For this review, use the dimensioned drawing (mm, ordinates from the lowest corner) and the shaded views. Coordinates: 2 decimals unless noted, no trailing zeros. Write each loop counter-clockwise with the first axis right and the second up, starting at its lowest first coordinate (ties: lowest second). Pieces come first, ordered by that corner, then holes. Notation, with made-up numbers: (41.25, 74.25) - (81.25, 74.25) arc R29 cw to (81.25, 103.25) - close; hole circle Ø9 at (9, 82). An arc over 180 degrees is marked (long way). One line per item, written item: value.
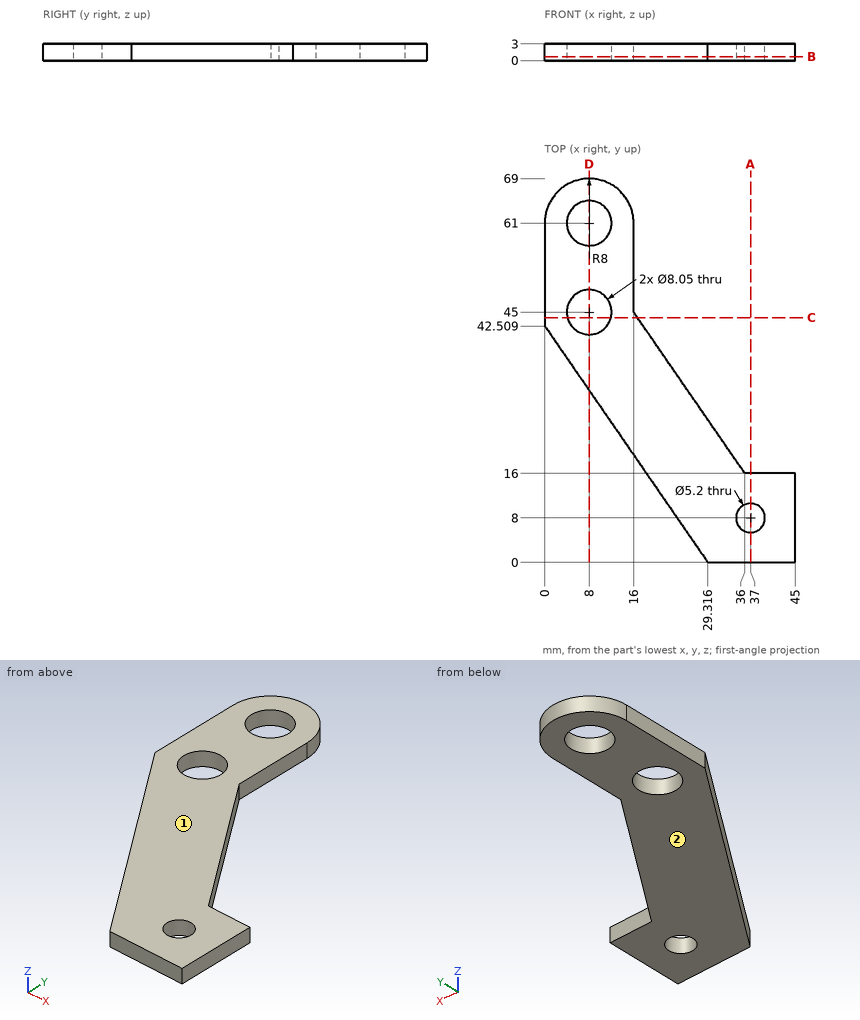
1. Consider section A-A, the plane x = 37. Write out the cut boundary in (y, z), then the cut area to 3 significant figures.
Answer block:
outline: (0, 0) - (5.4, 0) - (5.4, 3) - (0, 3) - close; (10.6, 0) - (16, 0) - (16, 3) - (10.6, 3) - close
area: 32.4 mm^2
2. Consider section D-D, the plane x = 8. Write out the cut boundary in (y, z) (1 decimal).
Answer block:
outline: (30.9, 0) - (41, 0) - (41, 3) - (30.9, 3) - close; (49, 0) - (57, 0) - (57, 3) - (49, 3) - close; (65, 0) - (69, 0) - (69, 3) - (65, 3) - close
3. Insertion check: pin 1 Ø1.5 at (x, z) = (27, 1) entering from +Y; pin 2 Ø1.5 at (y, z) = (43.5, 2) entering from +X; pin 3 Ø1 at (x, z) = (20.5, 2.5) entering from +Y; pin 4 Ø5 at (x, y) = (8, 61) entering from -Z. Each pin has a flat end and moves straight along its axis. Give the tip position at first contact, or say it passes through.
Answer block:
pin 1: stops at y = 30.14
pin 2: stops at x = 17.55
pin 3: stops at y = 39.2
pin 4: passes through
4. Mouldability with a two-part tool opening along Z and no side actions: class the marked faces 1 and 2 as released by +Z, released by -Z, zero draft, split by the parting line, or undercut.
Answer block:
face 1: released by +Z
face 2: released by -Z
5. Consider section B-B, the plane z = 0.75. Give the number of separate pieces and of enclosed holes in the cut face, then the cut area to 3 significant figures.
Answer block:
separate pieces: 1
enclosed holes: 3
area: 1,080 mm^2
6. Wall thickness on line 1 along Y through (x, z) = (37, 1.1); line 2 along Y through (x, z) = (4.5, 0.2) (1 decimal); line 3 along Y through (x, z) = (8, 1.1) (1 decimal): over which ranges is each line inside the solid? List them lowest first.
Answer block:
line 1: y = 0 to 5.4, 10.6 to 16
line 2: y = 36 to 43, 47 to 59, 63 to 68.2
line 3: y = 30.9 to 41, 49 to 57, 65 to 69
7. Consider section C-C, the plane y = 44. Write out the cut boundary in (x, z).
Answer block:
outline: (0, 0) - (4.1, 0) - (4.1, 3) - (0, 3) - close; (11.9, 0) - (16.69, 0) - (16.69, 3) - (11.9, 3) - close
